The model under review builds one solid part; all positions refer to its coordinate system, in mm. A direction names the side the tool comes from. Round coordinates to 2 decimals unless told otherwise and drop trailing zeros. Order: outer loops, then holes, each group sorted by start corner. A loop starts at its lowest first (then second) coordinate and runs counter-clockwise, first axis right, second up. Notation, with made-up numbers: (31, 52) -> (57, 52) arc R20 ccw to (57, 82) -> close; hole circle Ø8 at (-19.75, -40). An arc over 180 degrees is marked (long way). Put each result on its own line as item: value. Start each with the question number.
from build123d import *

# Parameters (mm, degrees)
SKETCH1_W           = 300
SKETCH1_H           = 420
BOSS_EXTRUDE1_DEPTH = 100
SKETCH2_W           = 240
SKETCH2_H           = 300
CUT_EXTRUDE1_DEPTH  = 20
SKETCH3_W           = 180
SKETCH3_H           = 240
BOSS_EXTRUDE2_DEPTH = 10
SKETCH4_W           = 30
SKETCH4_H           = 30
BOSS_EXTRUDE3_DEPTH = 5
FILLET1_R           = 5
FILLET2_R           = 5


with BuildPart() as part:
    # Sketch1 → Boss-Extrude1 (new body)
    with BuildSketch(Plane.XY):
        with Locations((150, 210)):
            Rectangle(SKETCH1_W, SKETCH1_H)
    extrude(amount=BOSS_EXTRUDE1_DEPTH)

    # Sketch2 → Cut-Extrude1 (cut)
    with BuildSketch(Plane.XY.offset(100)):
        with Locations((150, 210)):
            Rectangle(SKETCH2_W, SKETCH2_H)
    extrude(amount=-CUT_EXTRUDE1_DEPTH, mode=Mode.SUBTRACT)

    # Sketch3 → Boss-Extrude2 (add)
    with BuildSketch(Plane.XY.offset(80)):
        with Locations((150, 210)):
            Rectangle(SKETCH3_W, SKETCH3_H)
    extrude(amount=BOSS_EXTRUDE2_DEPTH)

    # Sketch4 → Boss-Extrude3 (add)
    with BuildSketch(Plane.XY.offset(90)):
        with Locations((91, 250)):
            Rectangle(SKETCH4_W, SKETCH4_H)
        with Locations((151, 250)):
            Rectangle(SKETCH4_W, SKETCH4_H)
        with Locations((183, 250)):
            Rectangle(SKETCH4_W, SKETCH4_H)
        with Locations((215, 250)):
            Rectangle(SKETCH4_W, SKETCH4_H)
        with Locations((87, 170)):
            Rectangle(SKETCH4_W, SKETCH4_H)
        with Locations((119, 170)):
            Rectangle(SKETCH4_W, SKETCH4_H)
        with Locations((151, 170)):
            Rectangle(SKETCH4_W, SKETCH4_H)
        with Locations((183, 170)):
            Rectangle(SKETCH4_W, SKETCH4_H)
        with Locations((215, 170)):
            Rectangle(SKETCH4_W, SKETCH4_H)
    extrude(amount=BOSS_EXTRUDE3_DEPTH)

    # Fillet1
    fillet1_edges = [part.edges().sort_by_distance(p)[0] for p in [
        (300, 210, 100),
        (150, 0, 100),
        (30, 210, 100),
        (150, 60, 100),
        (270, 210, 100),
        (150, 360, 100),
        (0, 210, 100),
        (150, 420, 100),
        (0, 0, 50),
        (300, 0, 50),
        (300, 420, 50),
        (0, 420, 50),
    ]]
    fillet(fillet1_edges, radius=FILLET1_R)

    # Fillet2
    fillet2_edges = [part.edges().sort_by_distance(p)[0] for p in [
        (150, 330, 90),
        (60, 210, 90),
        (150, 90, 90),
        (240, 210, 90),
    ]]
    fillet(fillet2_edges, radius=FILLET2_R)


solid = part.part
Q1. Wall thickness on probe 1 along Y at (x, z) = (210, 92); probe 2 along X at (y, z) = (298, 86); probe 3 along Z at (x, y) = (136, 230.5): over which ranges is each line inside the solid? List them lowest first. Write a range as [from, to].
Q2. Take a section at C-C on x = 264.5. Give the boundary of the cut face in (y, z).
Q3. For faces 1 (the face through (19, 213, 100)), 2 (the face through (183, 250, 95)), list the 3-axis set-ups (+Z, -Z, +X, -X, +Y, -Y) from which the entire face can be reached by the end or side of a thin tool; tool diameter is ignored.
Q4. Take a section at B-B on y = 319. Give the boundary of the cut face in (x, z), and give its area (3 significant figures).
Q5. Draft analysis for pull direction Y (two halves, no side actions). For faces 3 (the face through (300, 207, 47)), 4 (the face through (42, 212, 80)), 5 (the face through (148, 0, 47)), 6 (the face through (148, 420, 47)), state which applies: +Y half, -Y half, draft (parallel to the pull), parting line (faces both ways), or undercut.
Q6. Take a section at A-A on x = 151.5. Give the boundary of the cut face in (y, z), and give its area (3 significant figures).
Q7. Clearance check with a flat-ended pin moving along its axis: pin 1 Ø9 at (x, y) = (208.5, 252.5) entering from +Z. State where the tip first meets the part, or that it passes through.
Calculated:
1. probe 1: y = [0, 60], [155, 185], [235, 265], [360, 420]
1. probe 2: x = [0, 30], [60.1, 239.9], [270, 300]
1. probe 3: z = [0, 90]
2. outline: (0, 0) -> (420, 0) -> (420, 95) arc R5 ccw to (415, 100) -> (365, 100) arc R5 ccw to (360, 95) -> (360, 80) -> (60, 80) -> (60, 95) arc R5 ccw to (55, 100) -> (5, 100) arc R5 ccw to (0, 95) -> close
3. face 1: +Z, +X, -X, +Y, -Y
3. face 2: +Z
4. outline: (0, 0) -> (300, 0) -> (300, 95) arc R5 ccw to (295, 100) -> (275, 100) arc R5 ccw to (270, 95) -> (270, 80) -> (240, 80) -> (240, 85) arc R5 ccw to (235, 90) -> (65, 90) arc R5 ccw to (60, 85) -> (60, 80) -> (30, 80) -> (30, 95) arc R5 ccw to (25, 100) -> (5, 100) arc R5 ccw to (0, 95) -> close
4. area: 27,000 mm²
5. face 3: draft
5. face 4: undercut
5. face 5: -Y half
5. face 6: +Y half
6. outline: (0, 0) -> (420, 0) -> (420, 95) arc R5 ccw to (415, 100) -> (365, 100) arc R5 ccw to (360, 95) -> (360, 80) -> (330, 80) -> (330, 85) arc R5 ccw to (325, 90) -> (265, 90) -> (265, 95) -> (235, 95) -> (235, 90) -> (185, 90) -> (185, 95) -> (155, 95) -> (155, 90) -> (95, 90) arc R5 ccw to (90, 85) -> (90, 80) -> (60, 80) -> (60, 95) arc R5 ccw to (55, 100) -> (5, 100) arc R5 ccw to (0, 95) -> close
6. area: 38,700 mm²
7. pin 1: stops at z = 95
